CAD build for the part. Positions are in the model's coordinates, mm. A direction names the side the tool comes from. Round coordinates to 2 decimals unless told otherwise and drop trailing zeros. Loops run counter-clockwise (first coordinate to the right, second up) from the corner with the lowest first, then second, coordinate; pieces in that order, holes last.
```python
from build123d import *

# Parameters (mm, degrees)
F1_DEPTH = 30
F0_W     = 10
F0_H     = 30
F2_DEPTH = 30
F3_DEPTH = 30
F4_R     = 2
F5_DEPTH = 70.001


with BuildPart() as f1:
    # F0 (on Front) → F1 (new body)
    with BuildSketch(Plane.XZ):
        Polygon((-16, -4.3), (16, -4.3), (16, 4.3), (6, 4.3), (6, 34.3), (35, 34.3), (35, 45), (25, 45), (-25, 45), (-35, 45), (-35, 35), (-6, 35), (-6, 4.3), (-16, 4.3), align=None)
    extrude(amount=F1_DEPTH)

    # F0 (on Front) → F2 (join)
    with BuildSketch(Plane.XZ):
        with Locations((30, 60)):
            Rectangle(F0_W, F0_H)
    extrude(amount=F2_DEPTH)

    # F0 (on Front) → F3 (join)
    with BuildSketch(Plane.XZ):
        with Locations((-30, 60)):
            Rectangle(F0_W, F0_H)
    extrude(amount=F3_DEPTH)

    # F4 (on face) → F5 (cut, through all)
    with BuildSketch(Plane(origin=(-35, 0, 0), x_dir=(0, -1, 0), z_dir=(-1, 0, 0))):
        with Locations((15, 65)):
            Circle(F4_R)
    extrude(amount=-F5_DEPTH, mode=Mode.SUBTRACT)


solid = f1.part
```
Item 1: Cut at A-A, the plane y = -15. Give the cut face in (x, z), plus the area to 3 significant figures.
Answers follow:
outline: (-35, 35) - (-6, 35) - (-6, 4.3) - (-16, 4.3) - (-16, -4.3) - (16, -4.3) - (16, 4.3) - (6, 4.3) - (6, 34.3) - (35, 34.3) - (35, 63) - (25, 63) - (25, 45) - (-25, 45) - (-25, 63) - (-35, 63) - close; (-35, 67) - (-25, 67) - (-25, 75) - (-35, 75) - close; (25, 67) - (35, 67) - (35, 75) - (25, 75) - close
area: 1,880 mm2
Item 2: Cut at C-C, the plane z = 65. Give the cut face in (x, y).
Answers follow:
outline: (-35, -30) - (-25, -30) - (-25, -17) - (-35, -17) - close; (-35, -13) - (-25, -13) - (-25, 0) - (-35, 0) - close; (25, -30) - (35, -30) - (35, -17) - (25, -17) - close; (25, -13) - (35, -13) - (35, 0) - (25, 0) - close
Item 3: Cut at B-B, the plane x = 13.5. Give the cut face in (y, z).
Answers follow:
outline: (-30, -4.3) - (0, -4.3) - (0, 4.3) - (-30, 4.3) - close; (-30, 34.3) - (0, 34.3) - (0, 45) - (-30, 45) - close
Item 4: Probe line 1 (X direction, y = -5.25, z = 68.5); line 2 (Z direction, x = 29.5, y = -15); line 3 (Z direction, x = -29, y = -15). List the from-to ranges inside material, lowest first.
Answers follow:
line 1: x = -35 to -25, 25 to 35
line 2: z = 34.3 to 63, 67 to 75
line 3: z = 35 to 63, 67 to 75
Item 5: 3-axis set-ups, long thin cutter, end or side, ignore diameter. For faces 1 (the flat face through (0, -15, 45)), 2 (the flat face through (20, -15, 34.3)), 3 (the flat face through (-16, -15, 0)), 4 (the flat face through (-11, -15, 4.3)): which of +Z, -Z, +X, -X, +Y, -Y reach the whole face in a straight line?
Answers follow:
face 1: +Z, +Y, -Y
face 2: +X, +Y, -Y
face 3: -Z, -X, +Y, -Y
face 4: -X, +Y, -Y
Item 6: Two-plate mould, pull along X, no slides. Class faces 5 (the flat face through (16, -15, 0)), 6 (the cylindrical face through (30, -15, 67)), 7 (the flat face through (-25, -15, 60)), 8 (the flat face through (-6, -15, 20)): released by +X, released by -X, zero draft, split by the parting line, or undercut.
Answers follow:
face 5: released by +X
face 6: zero draft
face 7: undercut
face 8: released by -X
Item 7: Flat gauge pins, fed straight in: P1, Ø5, axis at x = 9.5, y = -16, coming from the +Z side; P2, Ø15, axis at y = -9.5, z = 18.5, coming from the +X side; P3, Ø9.5, axis at y = -20, z = 1.5, coming from the +X side; P4, Ø2.5, axis at y = -15, z = 65, coming from the -X side. Where does each tip first touch, or does it go through?
Answers follow:
P1: stops at z = 45
P2: stops at x = 6
P3: stops at x = 16
P4: passes through
Item 8: Cut at D-D, the plane y = -25.75. Give the cut face in (x, z), plus the area to 3 significant figures.
Answers follow:
outline: (-35, 35) - (-6, 35) - (-6, 4.3) - (-16, 4.3) - (-16, -4.3) - (16, -4.3) - (16, 4.3) - (6, 4.3) - (6, 34.3) - (35, 34.3) - (35, 75) - (25, 75) - (25, 45) - (-25, 45) - (-25, 75) - (-35, 75) - close
area: 1,960 mm2
